Read the model definition and answer for the solid it produces. Units are mm, in the model's axes. A direction names the side the tool comes from. Give positions to 0.01 mm unless a question says otherwise; leave off trailing zeros. Write each loop counter-clockwise with the first axis right and the second up, starting at its lowest first coordinate (ties: lowest second). Pieces come first, ordered by that corner, then holes. Notation, with made-up numbers: M 32.25,11 L 39.25,11 A7 cw 39.25,22 Z; hole C 75.25,-11 d2. An arc over 180 degrees is marked long. Use a Markdown table: item, result. Add a question column.
Item 1: A cutting plane is placed at B-B on x = 0. Determine the outline of the cut face in (y, z), then the cut area to 3 significant figures.
Item 2: Given P1, Ø1, axis at x = -39, y = 1, coming from the +Z side; P2, Ø1.5, axis at x = 32.5, y = 1, coming from the +Z side; P3, Ø1, axis at x = -69, y = 3, coming from the -Z side, each flat-ended and moving along its own axis, determine where each tip first touches the part or whether it passes through.
Item 3: A cutting plane is placed at C-C on y = 2.9. Determine the outline of the cut face in (x, z), then the cut area to 3 significant figures.
Item 4: The mould has two halves that part along X. Classify faces 3 (the cylindrical face through (-134.91, 1.77, 103.44)), 4 (the cylindrical face through (-19.527, 0.74, -148.724)), 5 (the flat face through (-81, 1.5, -127)), 6 (the flat face through (-0.8, 0, 150.3)): pulls with the +X half, pulls with the -X half, needs draft (parallel to the pull), parting line crosses it, or undercut.
Item 5: Consider probe 1 along X at (y, z) = (0.9, 0); probe 2 along X at (y, z) = (2, 0); probe 3 along Z at (x, y) = (3, 0.55). Determine where each line is inside the solid, lowest interval first. Write a range as [from, to].
Item 6: For faces 1 (the flat face through (150.3, 3.5, -38.6)), 2 (the cylindrical face through (-33.601, 2.514, 151.314)), determine the directions among +Z, -Z, +X, -X, +Y, -Y from which every point of the face is accessible in a straight line to the end or side of a thin tool.
Item 7: A cutting plane is placed at A-A on z = 0. Determine the outline of the cut face in (x, y).
from build123d import *

# Parameters (mm, degrees)
SKETCH_1_R          = 160
SKETCH_1_R_2        = 150
EXTRUDE_1_DEPTH     = 1.5
SKETCH_2_R          = 160
SKETCH_2_R_2        = 152.5
EXTRUDE_2_DEPTH     = 2
SKETCH_3_R          = 170
SKETCH_3_R_2        = 160
EXTRUDE_3_DEPTH     = 3.5
SKETCH_4_R          = 155
SKETCH_4_R_2        = 152.5
CUT_EXTRUDE_1_DEPTH = 2


with BuildPart() as part:
    # ｽｹｯﾁ1 → ﾎﾞｽ - 押し出し1 (new body)
    with BuildSketch(Plane(origin=(0, 0, 0), x_dir=(1, 0, 0), z_dir=(0, 1, 0))):
        Circle(SKETCH_1_R)
        Circle(SKETCH_1_R_2, mode=Mode.SUBTRACT)
    extrude(amount=EXTRUDE_1_DEPTH)

    # ｽｹｯﾁ2 → ﾎﾞｽ - 押し出し2 (add)
    with BuildSketch(Plane(origin=(0, 1.5, 0), x_dir=(1, 0, 0), z_dir=(0, 1, 0))):
        Circle(SKETCH_2_R)
        Circle(SKETCH_2_R_2, mode=Mode.SUBTRACT)
    extrude(amount=EXTRUDE_2_DEPTH)

    # ｽｹｯﾁ3 → ﾎﾞｽ - 押し出し3 (add)
    with BuildSketch(Plane(origin=(0, 3.5, 0), x_dir=(1, 0, 0), z_dir=(0, 1, 0))):
        Circle(SKETCH_3_R)
        Circle(SKETCH_3_R_2, mode=Mode.SUBTRACT)
    extrude(amount=-EXTRUDE_3_DEPTH)

    # ｽｹｯﾁ4 → ｶｯﾄ - 押し出し1 (cut)
    with BuildSketch(Plane(origin=(0, 3.5, 0), x_dir=(1, 0, 0), z_dir=(0, 1, 0))):
        Circle(SKETCH_4_R)
        Circle(SKETCH_4_R_2, mode=Mode.SUBTRACT)
    extrude(amount=-CUT_EXTRUDE_1_DEPTH, mode=Mode.SUBTRACT)


solid = part.part
Filled in:
| question | item | result |
|---|---|---|
| 1 | outline | M 0,-170 L 3.5,-170 L 3.5,-155 L 1.5,-155 L 1.5,-150 L 0,-150 Z; M 0,150 L 1.5,150 L 1.5,155 L 3.5,155 L 3.5,170 L 0,170 Z |
| 1 | area | 120 mm² |
| 2 | P1 | z = 165.58 |
| 2 | P2 | z = 167.01 |
| 2 | P3 | z = -155.59 |
| 3 | outline | C 0,0 d340; hole C 0,0 d310 |
| 3 | area | 15,300 mm² |
| 4 | face 3 | parting line crosses it |
| 4 | face 4 | undercut |
| 4 | face 5 | undercut |
| 4 | face 6 | needs draft |
| 5 | probe 1 | [-170, -150], [150, 170] |
| 5 | probe 2 | [-170, -155], [155, 170] |
| 5 | probe 3 | [-169.97, -149.97], [149.97, 169.97] |
| 6 | face 1 | +Z, -Z, +X, -X, +Y |
| 6 | face 2 | +Y |
| 7 | outline | M -170,0 L -150,0 L -150,1.5 L -155,1.5 L -155,3.5 L -170,3.5 Z; M 150,0 L 170,0 L 170,3.5 L 155,3.5 L 155,1.5 L 150,1.5 Z |
